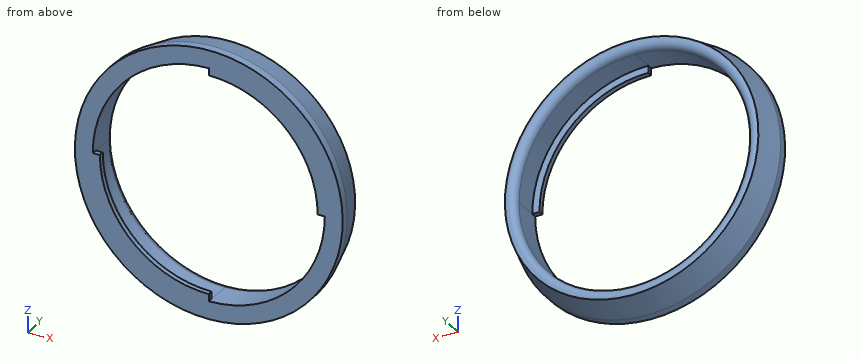
```python
from build123d import *

# Parameters (mm, degrees)
CUT_EXTRUDE2_DEPTH = 11.0000001


with BuildPart() as part:
    # Sketch1 → Revolve1 (revolve)
    with BuildSketch(Plane.XY, mode=Mode.PRIVATE) as revolve1_sk:
        with BuildLine():
            Line((37.5, 0), (30.5, 0))
            Line((30.5, 0), (30.5, 1.45))
            Line((30.5, 1.45), (32.5, 1.45))
            Line((32.5, 1.45), (32.5, 8))
            ThreePointArc((32.5, 8), (33.5, 9.732050808), (35.5, 9.732050808))
            Line((35.5, 9.732050808), (37.5, 2.267949192))
            Line((37.5, 2.267949192), (37.5, 0))
        make_face()
    revolve(revolve1_sk.sketch.rotate(Axis((0, 0, 0), (0, 1, 0)), 90), axis=Axis((0, 0, 0), (0, 1, 0)))  # turned: the seam where the file's is

    # Sketch2 → Cut-Extrude2 (cut, through all)
    with BuildSketch(Plane(origin=(0, 0, 0), x_dir=(1, 0, 0), z_dir=(0, 1, 0))):
        with BuildLine():
            Line((0, 30.5), (0, 32.5))
            ThreePointArc((0, 32.5), (22.980970389, 22.980970389), (32.5, 0))
            Line((32.5, 0), (30.5, 0))
            ThreePointArc((30.5, 0), (21.566756826, 21.566756826), (0, 30.5))
        make_face()
        with BuildLine():
            Line((0, -32.5), (0, -30.5))
            ThreePointArc((0, -30.5), (-21.566756826, -21.566756826), (-30.5, 0))
            Line((-30.5, 0), (-32.5, 0))
            ThreePointArc((-32.5, 0), (-22.980970389, -22.980970389), (0, -32.5))
        make_face()
    extrude(amount=CUT_EXTRUDE2_DEPTH, mode=Mode.SUBTRACT)


solid = part.part
```
CAD build for the part. Positions are in the model's coordinates, mm. Round coordinates to 2 decimals unless told otherwise and drop trailing zeros. Order: outer loops, then holes, each group sorted by start corner. A loop starts at its lowest first (then second) coordinate and runs counter-clockwise, first axis right, second up.
Q1. Drop flat-ended pins along their axis: pin 1 (1.2 mm diameter, centred on x = 31, y = 0.5, fed in from -Z); pin 2 (5 mm diameter, centred on y = 5.5, z = -19, fed in from +X); pin 3 (4 mm diameter, centred on y = 1.5, z = -27.5, fed in from +X); pin 4 (16.5 mm diameter, centred on x = -21.5, z = -21.5, fed in from +Y). Give the stop position or say it passes through.
Q2. Slice it at A-A (y = 6). Write the cut outline in (x, z), and give its area (3 significant figures).
Q3. Wall check: L1, parallel to Z at x = -1, y = 1.75; L2, parallel to Y at x = 31.5, z = 13.5; L3, parallel to Z at x = -20.5, y = 3.25. Give the ranges that are in metal, low to high.
Results below:
1. pin 1: stops at z = -21.96
1. pin 2: stops at x = 32.91
1. pin 3: stops at x = 27.5
1. pin 4: stops at y = 10
2. outline: circle Ø73 at (0, 0); hole circle Ø65 at (0, 0)
2. area: 867 mm2
3. L1: z = -37.49 to -32.48, 32.48 to 37.49
3. L2: y = 0 to 9.99
3. L3: z = -31.09 to -25.22, 25.22 to 31.09
